from build123d import *

# Parameters (mm, degrees)
SKETCH1_R           = 5.5
BOSS_EXTRUDE1_DEPTH = 5
SKETCH2_R           = 5
CUT_EXTRUDE1_DEPTH  = 3.9
CUT_EXTRUDE2_REACH  = 7
SKETCH3_R           = 4
SKETCH4_OUTSIDE_W   = 16.268
SKETCH4_OUTSIDE_H   = 16.268
SKETCH4_OUTSIDE_R   = 5.45
CUT_EXTRUDE3_DEPTH  = 2.5


with BuildPart() as part:
    # Sketch1 → Boss-Extrude1 (new body)
    with BuildSketch(Plane.XY):
        Circle(SKETCH1_R)
    extrude(amount=-BOSS_EXTRUDE1_DEPTH)

    # Sketch2 → Cut-Extrude1 (cut)
    with BuildSketch(Plane(origin=(0, 0, -5), x_dir=(-1, 0, 0), z_dir=(0, 0, -1))):
        Circle(SKETCH2_R)
    extrude(amount=-CUT_EXTRUDE1_DEPTH, mode=Mode.SUBTRACT)

    # Sketch3 → Cut-Extrude2 (cut, up to next)
    with BuildSketch(Plane.XY, mode=Mode.PRIVATE) as cut_extrude2_sk1:
        Circle(SKETCH3_R)
    cut_extrude2_tool1 = extrude(cut_extrude2_sk1.sketch, amount=-CUT_EXTRUDE2_REACH, mode=Mode.PRIVATE) & part.part
    add(cut_extrude2_tool1.solids().sort_by_distance((0, 0, 0))[0], mode=Mode.SUBTRACT)

    # Sketch4 outside → Cut-Extrude3 (cut)
    with BuildSketch(Plane.XY):
        Rectangle(SKETCH4_OUTSIDE_W, SKETCH4_OUTSIDE_H)
        Circle(SKETCH4_OUTSIDE_R, mode=Mode.SUBTRACT)
    extrude(amount=-CUT_EXTRUDE3_DEPTH, mode=Mode.SUBTRACT)


solid = part.part
Input: part model. Units: mm. Frame: model coordinates. Give positions to 0.01 mm unless a question says otherwise; leave off trailing zeros. Write each loop counter-clockwise with the first axis right and the second up, starting at its lowest first coordinate (ties: lowest second). Pieces come first, ordered by that corner, then holes.
Q1. Material intervals for probe 1 along Y at (x, z) = (0, -2.35); probe 2 along Y at (x, z) = (0, -3.85); probe 3 along X at (y, z) = (4.5, -2.95), sorted ascending.
Q2. Pull-direction query (Y, two-part tool) for faces 1 (the face through (5.198, 1.637, -1.232)), 2 (the face through (1.6, -4.9, -5)), 3 (the face through (1.08, -4.88, -3.08)); classes: pulls with the +Y half, pulls with the -Y half, needs draft (parallel to the pull), parting line crosses it, or undercut.
Q3. Section C-C, the plane z = -2. Output: boundary loops of the cut face in (x, y), plus the area to 3 significant figures.
Q4. First-contact query: P1, Ø1, axis at y = 1.5, z = -1.5, coming from the +X side; P2, Ø1.5, axis at x = 2, y = 3, coming from the -Z side; P3, Ø1.5, axis at x = -1.5, z = -2.5, coming from the +Y side. Flat tips, straight axial feed; report the tip coordinate or a pass-through.
Q5. Section D-D, the plane z = -4.2. Output: boundary loops of the cut face in (x, y).
Q6. Section A-A, the plane x = 0. Output: boundary loops of the cut face in (y, z), plus the area to 3 significant figures.
Filled in:
1. probe 1: y = -5.45 to -5, 5 to 5.45
1. probe 2: y = -5.5 to -5, 5 to 5.5
1. probe 3: x = -3.16 to -2.18, 2.18 to 3.16
2. face 1: parting line crosses it
2. face 2: needs draft
2. face 3: undercut
3. outline: circle Ø10.9 at (0, 0); hole circle Ø10 at (0, 0)
3. area: 14.8 mm2
4. P1: stops at x = 5.36
4. P2: stops at z = -1.1
4. P3: stops at y = 5.45
5. outline: circle Ø11 at (0, 0); hole circle Ø10 at (0, 0)
6. outline: (-5.5, -5) - (-5, -5) - (-5, -1.1) - (-4, -1.1) - (-4, 0) - (-5.45, 0) - (-5.45, -2.5) - (-5.5, -2.5) - close; (4, -1.1) - (5, -1.1) - (5, -5) - (5.5, -5) - (5.5, -2.5) - (5.45, -2.5) - (5.45, 0) - (4, 0) - close
6. area: 6.95 mm2
